Read the model definition and answer for the solid it produces. Units are mm, in the model's axes. A direction names the side the tool comes from. Round coordinates to 2 decimals unless told otherwise and drop trailing zeros. Order: outer loops, then holes, each group sorted by start corner. A loop starts at its lowest first (then second) coordinate and runs counter-clockwise, first axis right, second up. Notation, with made-up numbers: (-36.5, 84.25) -> (-7.5, 84.25) arc R35 ccw to (-7.5, 116.25) -> close; hole circle Ø7 at (13, -14). An arc over 180 degrees is marked (long way). Use a Markdown table: item, result. Add a question column.
1. Section C-C, the plane y = -15.5 is taken. Give the vertices of the cut face in (x, z), then the cut area to 3 significant figures.
2. For faces 1 (the face through (8.521, -22.554, -2.683)), 2 (the face through (28.575, 1, 0)), determine the directions among +Z, -Z, +X, -X, +Y, -Y from which every point of the face is accessible in a straight line to the end or side of a thin tool.
3. Given pin 1 (6 mm diameter, centred on y = -38, z = 0, fed in from -X); pin 2 (3 mm diameter, centred on x = 19.685, z = 0, fed in from -Y); pin 3 (12 mm diameter, centred on y = -20.5, z = -7, fed in from -X); pin 4 (1.5 mm diameter, centred on x = 3, y = -35, fed in from +Z), each flat-ended and moving along its own axis, determine where each tip first touches the part or whether it passes through.
4. Consider L1, parallel to X at y = 0.8, z = 0 (3 decimals); L2, parallel to X at y = 1.3, z = 0 (3 decimals); L3, parallel to Z at x = -6, y = -12. Determine where each line is inside the solid, lowest interval first. Write a range as [from, to].
5. Section B-B, the plane x = 14 is taken. Give the vertices of the cut face in (y, z), then the cut area to 3 significant figures.
6. The mould has two halves that part along X. Classify faces 3 (the face through (-17.572, 1.252, -1.099)), 4 (the face through (26.764, 1.252, -10.79)), 5 (the face through (-28.575, 1, 0)), 6 (the face through (-4.38, -23.87, -10.57)): +X half, -X half, draft (parallel to the pull), parting line (faces both ways), or undercut.
7. Section A-A, the plane z = 0 is taken. Give the number of separate pieces and of enclosed holes in the cut face, then the cut area to 3 significant figures.
8. Section D-D, the plane y = -40 is taken. Give the vertices of the cut face in (x, z).
```python
from build123d import *

# Parameters (mm, degrees)
BOSS_EXTRUDE1_DEPTH = 2.54
SKETCH2_R           = 12.065
BOSS_EXTRUDE2_DEPTH = 54.61
DRAFT2_ANGLE        = 1.5
FILLET2_R           = 6.35
CUT_EXTRUDE1_REACH  = 64.929
SKETCH3_R           = 2.38125


# Read off the part's stored shape, not the designer's step: Shell1
with BuildPart() as part:
    # Sketch1 → Boss-Extrude1 (new body)
    with BuildSketch(Plane(origin=(0, 0, 0), x_dir=(1, 0, 0), z_dir=(0, 1, 0))):
        with BuildLine():
            Line((-22.225, -12.7), (22.225, -12.7))
            ThreePointArc((22.225, -12.7), (26.715128061, -10.840128061), (28.575, -6.35))
            Line((28.575, -6.35), (28.575, 6.35))
            ThreePointArc((28.575, 6.35), (26.715128061, 10.840128061), (22.225, 12.7))
            Line((22.225, 12.7), (-22.225, 12.7))
            ThreePointArc((-22.225, 12.7), (-26.715128061, 10.840128061), (-28.575, 6.35))
            Line((-28.575, 6.35), (-28.575, -6.35))
            ThreePointArc((-28.575, -6.35), (-26.715128061, -10.840128061), (-22.225, -12.7))
        make_face()
    extrude(amount=BOSS_EXTRUDE1_DEPTH)

    # Sketch2 → Boss-Extrude2 (add)
    with BuildSketch(Plane.XZ):
        with Locations(Location((0, 0, 0), (0, 0, 270))):
            Circle(SKETCH2_R)
    extrude(amount=BOSS_EXTRUDE2_DEPTH)

    # Draft2
    draft2_faces = [part.faces().sort_by_distance(p)[0] for p in [
        (0, -27.305, 12.065),
    ]]
    draft(draft2_faces, Plane(origin=(22.225, 0, 6.35), x_dir=(0, 0, -1), z_dir=(0, -1, 0)), DRAFT2_ANGLE)

    # Fillet2
    fillet2_edges = [part.edges().sort_by_distance(p)[0] for p in [
        (0, -54.61, 10.634986823),
    ]]
    fillet(fillet2_edges, radius=FILLET2_R)

    # Shell1 outline → Shell1 (revolve, cut)
    with BuildSketch(Plane.XY):
        with BuildLine():
            ThreePointArc((4.449090693, -52.07), (7.107672345, -50.989110404), (8.257785101, -48.359734173))
            Line((8.257785101, -48.359734173), (9.590641548, 2.54))
            Line((9.590641548, 2.54), (0, 2.54))
            Line((0, 2.54), (0, -52.07))
            Line((0, -52.07), (4.449090693, -52.07))
        make_face()
    revolve(axis=Axis((0, 0, 0), (0, 1, 0)), mode=Mode.SUBTRACT)

    # Sketch3 → Cut-Extrude1 (cut, up to next)
    with BuildSketch(Plane.XZ, mode=Mode.PRIVATE) as cut_extrude1_sk1:
        with Locations(Location((19.685, 0, 0), (0, 0, 270))):
            Circle(SKETCH3_R)
    cut_extrude1_tool1 = extrude(cut_extrude1_sk1.sketch, amount=-CUT_EXTRUDE1_REACH, mode=Mode.PRIVATE) & part.part
    cut_extrude1 = cut_extrude1_tool1.solids().sort_by_distance((19.685, 0, 0))[0]
    add(cut_extrude1, mode=Mode.SUBTRACT)

    # Mirror1: Cut-Extrude1 across plane
    add(cut_extrude1.mirror(Plane(origin=(0, 0, 0), x_dir=(0, 0, 1), z_dir=(1, 0, 0))), mode=Mode.SUBTRACT)


solid = part.part
```
Verdict:
| question | item | result |
|---|---|---|
| 1 | outline | circle Ø23.32 at (0, 0); hole circle Ø18.24 at (0, 0) |
| 1 | area | 166 mm2 |
| 2 | face 1 | +Y |
| 2 | face 2 | +Z, -Z, +X, +Y, -Y |
| 3 | pin 1 | stops at x = -11.15 |
| 3 | pin 2 | passes through |
| 3 | pin 3 | stops at x = -11.51 |
| 3 | pin 4 | stops at z = 10.92 |
| 4 | L1 | x = [-28.575, -22.066], [-17.304, -9.545], [9.545, 17.304], [22.066, 28.575] |
| 4 | L2 | x = [-28.575, -22.066], [-17.304, -9.558], [9.558, 17.304], [22.066, 28.575] |
| 4 | L3 | z = [-10.1, -6.99], [6.99, 10.1] |
| 5 | outline | (0, -12.7) -> (2.54, -12.7) -> (2.54, 12.7) -> (0, 12.7) -> close |
| 5 | area | 64.5 mm2 |
| 6 | face 3 | undercut |
| 6 | face 4 | +X half |
| 6 | face 5 | -X half |
| 6 | face 6 | parting line |
| 7 | separate pieces | 3 |
| 7 | enclosed holes | 0 |
| 7 | area | 381 mm2 |
| 8 | outline | circle Ø22.04 at (0, 0); hole circle Ø16.95 at (0, 0) |
